from build123d import *

# Parameters (mm, degrees)
WALL_MOUNTING_PLATE_4MM_START        = 68
SKETCH1_W                            = 36
SKETCH1_H                            = 110
WALL_MOUNTING_PLATE_4MM_DEPTH        = 4
SIDE_OFFSET_WEB_START                = 44.3
SKETCH2_W                            = 4
SKETCH2_H                            = 86
SIDE_OFFSET_WEB_DEPTH                = 24
TWO_PEG_RECEIVER_TABS_START          = 44.3
SKETCH3_W                            = 32
SKETCH3_H                            = 24
TWO_PEG_RECEIVER_TABS_DEPTH          = 3.2
PEG_HEAD_ENTRY_D9P8_START            = 43
SKETCH4_R                            = 4.9
PEG_HEAD_ENTRY_D9P8_DEPTH            = 9
DROP_IN_PEG_SLOTS_W5P8_START         = 43
SKETCH5_W                            = 5.8
SKETCH5_H                            = 8.6
DROP_IN_PEG_SLOTS_W5P8_DEPTH         = 9
ROUNDED_LOAD_SEATS_START             = 43
SKETCH6_R                            = 2.9
ROUNDED_LOAD_SEATS_DEPTH             = 9
WALL_SCREW_CLEARANCE_D5P5_START      = 67
SKETCH7_R                            = 2.75
WALL_SCREW_CLEARANCE_D5P5_DEPTH      = 7
ANTI_LIFT_LOCK_TAB_START             = 44.3
SKETCH8_W                            = 25
SKETCH8_H                            = 10
ANTI_LIFT_LOCK_TAB_DEPTH             = 3.2
ANTI_LIFT_SCREW_CLEARANCE_D3P4_START = 43
SKETCH9_R                            = 1.7
ANTI_LIFT_SCREW_CLEARANCE_D3P4_DEPTH = 7


with BuildPart() as part:
    # Sketch1 → Wall_mounting_plate_4mm (new body)
    with BuildSketch(Plane.XY.offset(WALL_MOUNTING_PLATE_4MM_START)):
        with Locations((-20, 0)):
            Rectangle(SKETCH1_W, SKETCH1_H)
    extrude(amount=WALL_MOUNTING_PLATE_4MM_DEPTH)

    # Sketch2 → Side_offset_web (add)
    with BuildSketch(Plane.XY.offset(SIDE_OFFSET_WEB_START)):
        with Locations((-36, 0)):
            Rectangle(SKETCH2_W, SKETCH2_H)
    extrude(amount=SIDE_OFFSET_WEB_DEPTH)

    # Sketch3 → Two_peg_receiver_tabs (add)
    with BuildSketch(Plane.XY.offset(TWO_PEG_RECEIVER_TABS_START)):
        with Locations((-22, -28)):
            Rectangle(SKETCH3_W, SKETCH3_H)
        with Locations((-22, 22)):
            Rectangle(SKETCH3_W, SKETCH3_H)
    extrude(amount=TWO_PEG_RECEIVER_TABS_DEPTH)

    # Sketch4 → Peg_head_entry_D9p8 (cut)
    with BuildSketch(Plane.XY.offset(PEG_HEAD_ENTRY_D9P8_START)):
        with Locations((-20, -34)):
            Circle(SKETCH4_R)
        with Locations((-20, 16)):
            Circle(SKETCH4_R)
    extrude(amount=PEG_HEAD_ENTRY_D9P8_DEPTH, mode=Mode.SUBTRACT)

    # Sketch5 → Drop_in_peg_slots_W5p8 (cut)
    with BuildSketch(Plane.XY.offset(DROP_IN_PEG_SLOTS_W5P8_START)):
        with Locations((-20, -29.7)):
            Rectangle(SKETCH5_W, SKETCH5_H)
        with Locations((-20, 20.3)):
            Rectangle(SKETCH5_W, SKETCH5_H)
    extrude(amount=DROP_IN_PEG_SLOTS_W5P8_DEPTH, mode=Mode.SUBTRACT)

    # Sketch6 → Rounded_load_seats (cut)
    with BuildSketch(Plane.XY.offset(ROUNDED_LOAD_SEATS_START)):
        with Locations((-20, -25.4)):
            Circle(SKETCH6_R)
        with Locations((-20, 24.6)):
            Circle(SKETCH6_R)
    extrude(amount=ROUNDED_LOAD_SEATS_DEPTH, mode=Mode.SUBTRACT)

    # Sketch7 → Wall_screw_clearance_D5p5 (cut)
    with BuildSketch(Plane.XY.offset(WALL_SCREW_CLEARANCE_D5P5_START)):
        with Locations((-20, -45)):
            Circle(SKETCH7_R)
        with Locations((-20, 45)):
            Circle(SKETCH7_R)
    extrude(amount=WALL_SCREW_CLEARANCE_D5P5_DEPTH, mode=Mode.SUBTRACT)

    # Sketch8 → Anti_lift_lock_tab (add)
    with BuildSketch(Plane.XY.offset(ANTI_LIFT_LOCK_TAB_START)):
        with Locations((-25.5, 0)):
            Rectangle(SKETCH8_W, SKETCH8_H)
    extrude(amount=ANTI_LIFT_LOCK_TAB_DEPTH)

    # Sketch9 → Anti_lift_screw_clearance_D3p4 (cut)
    with BuildSketch(Plane.XY.offset(ANTI_LIFT_SCREW_CLEARANCE_D3P4_START)):
        with Locations((-20, 0)):
            Circle(SKETCH9_R)
    extrude(amount=ANTI_LIFT_SCREW_CLEARANCE_D3P4_DEPTH, mode=Mode.SUBTRACT)


solid = part.part
Design review of the part built by this model. Coordinates are the model's own, in mm. A direction names the side the tool comes from. Give positions to 0.01 mm unless a question says otherwise; leave off trailing zeros. Write each loop counter-clockwise with the first axis right and the second up, starting at its lowest first coordinate (ties: lowest second). Pieces come first, ordered by that corner, then holes. Notation, with made-up numbers: M -30,1.5 L 25,1.5 A24 cw 25,23.5 Z; hole C -28,41.25 d8. An arc over 180 degrees is marked long. Return JSON: item names as keys, results as strings. Group by question number.
Item 1: Take a section at C-C (y = 0). Give the boundary of the cut face in (x, z).
Item 2: Take a section at A-A (y = -34). Give the boundary of the cut face in (x, z), plus the area to 3 significant figures.
Item 3: The part is to be moulded in two halves that separate along Z. For faces 4 (the flat face through (-20, 1, 72)), 5 (the flat face through (-20, 1, 68)), 6 (the flat face through (-24, 0, 47.5)), 7 (the cylindrical face through (-20.358, 47.727, 69.972)), say which applies: pulls with the +Z half, pulls with the -Z half, needs draft (parallel to the pull), parting line crosses it, or undercut.
Item 4: Clearance check with flat-ended pins moving along their axes: pin 1 Ø1 at (y, z) = (0.5, 46.5) entering from +X; pin 2 Ø1 at (y, z) = (24.5, 45.5) entering from +X; pin 3 Ø2.5 at (x, z) = (-19.5, 45.5) entering from -Y; pin 4 Ø4.5 at (x, y) = (-20, 45) entering from -Z. State where each tip first meets the part, or that it passes through.
Item 5: Wall thickness on line 1 along Y through (x, z) = (-20, 45.6); line 2 along Y through (x, z) = (-20, 70.8); line 3 along X through (y, z) = (45, 70.05): over which ranges is each line inside the solid? List them lowest first.
Item 6: Take a section at D-D (z = 59.5). Give the boundary of the cut face in (x, y), plus the area to 3 significant figures.
Item 7: Take a section at B-B (x = -20). Count the separate pieces of the cut face and the enclosed holes in it, plus the area to 3 significant figures.
Item 8: Tool access review of faces 1 (the cylindrical face through (-18.43, -0.65, 45.88)), 2 (the flat face through (-6, -28, 46)), 3 (the flat face through (-20, -16, 46)): name each direction out of +Z, -Z, +X, -X, +Y, -Y from which nothing blocks a thin tool from reaching the whole face with its end or side.
Return value:
{
 "1": {"outline": "M -38,44.3 L -21.7,44.3 L -21.7,47.5 L -34,47.5 L -34,68 L -2,68 L -2,72 L -38,72 Z; M -18.3,44.3 L -13,44.3 L -13,47.5 L -18.3,47.5 Z"},
 "2": {"outline": "M -38,44.3 L -24.9,44.3 L -24.9,47.5 L -34,47.5 L -34,68 L -2,68 L -2,72 L -38,72 Z; M -15.1,44.3 L -6,44.3 L -6,47.5 L -15.1,47.5 Z", "area": "297 mm2"},
 "3": {"face 4": "pulls with the +Z half", "face 5": "undercut", "face 6": "undercut", "face 7": "needs draft"},
 "4": {"pin 1": "stops at x = -13", "pin 2": "stops at x = -6", "pin 3": "stops at y = -40", "pin 4": "passes through"},
 "5": {"line 1": "y = -40 to -38.9, -22.5 to -16, -5 to -1.7, 1.7 to 5, 10 to 11.1, 27.5 to 34", "line 2": "y = -55 to -47.75, -42.25 to 42.25, 47.75 to 55", "line 3": "x = -38 to -22.75, -17.25 to -2"},
 "6": {"outline": "M -38,-43 L -34,-43 L -34,43 L -38,43 Z", "area": "344 mm2"},
 "7": {"separate pieces": "9", "enclosed holes": "0", "area": "466 mm2"},
 "8": {"face 1": "-Z", "face 2": "-Z, +X, +Y, -Y", "face 3": "-Z, +X"}
}
